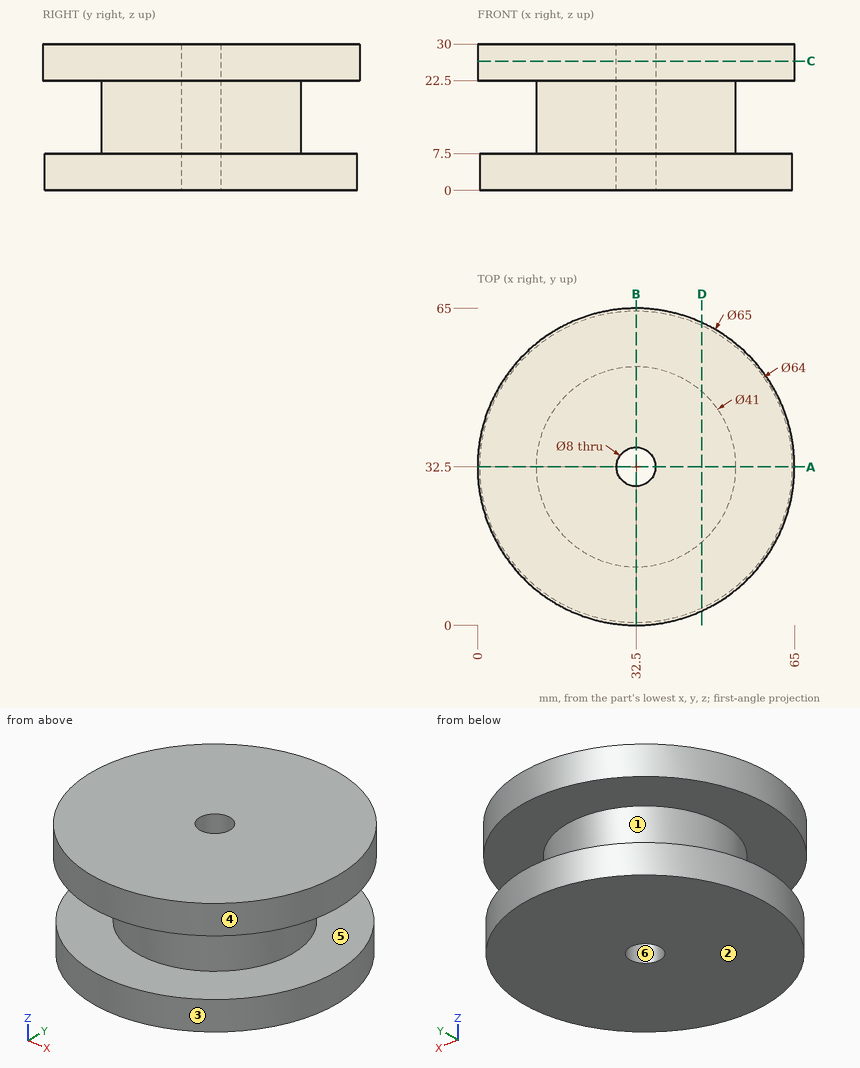
For this review, use the dimensioned drawing (mm, ordinates from the lowest corner) and the shaded views. A direction names the side the tool comes from. Give positions to 0.01 mm unless a question says otherwise; leave off trailing zeros. Order: outer loops, then holes, each group sorted by start corner. A loop starts at its lowest first (then second) coordinate and runs counter-clockwise, first axis right, second up. Notation, with made-up numbers: (-10, 37.25) - (-6, 37.25) arc R14 ccw to (-6, 41.25) - close; hole circle Ø4 at (21, -17.5). An arc over 180 degrees is marked (long way). Write item = value, one per line. Start each with the question number.
Q1. We need section A-A on y = 32.5. State the section outline as (x, z) points.
Q2. To check wall thickness, follow L1, parallel to Z at x = 11, y = 23.5; L2, parallel to Y at x = 32.5, z = 11.75; L3, parallel to Z at x = 19.5, y = 62. State the ranges of each line that lie inside material, in increasing order. Write a range as from..to.
Q3. We need section D-D on x = 46. State the section outline as (y, z) points.
Q4. We need section C-C on z = 26.5. State the section outline as (x, y) points, plus the area to 3 significant figures.
Q5. Clearance check with flat-ended pins moving along their axes: pin 1 Ø3 at (x, z) = (53.5, 24) entering from -Y; pin 2 Ø12 at (x, z) = (16.5, 19.5) entering from +Y; pin 3 Ø2 at (y, z) = (20, 4) entering from +X; pin 4 Ø10 at (x, y) = (45, 17.5) entering from -Z. State where each tip first meets the part, or that it passes through.
Q6. Tool access review of the marked faces 1, 2 and 3: name each direction out of +Z, -Z, +X, -X, +Y, -Y from which nothing blocks a thin tool from reaching the whole face with its end or side.
Q7. Mouldability with a two-part tool opening along X and no side actions: class the marked faces 4, 5 and 6 as released by +X, released by -X, zero draft, split by the parting line, or undercut.
Working result:
q1.outline = (0, 22.5) - (12, 22.5) - (12, 7.5) - (0.5, 7.5) - (0.5, 0) - (28.5, 0) - (28.5, 30) - (0, 30) - close; (36.5, 0) - (64.5, 0) - (64.5, 7.5) - (53, 7.5) - (53, 22.5) - (65, 22.5) - (65, 30) - (36.5, 30) - close
q2.L1 = 0..7.5, 22.5..30
q2.L2 = 12..28.5, 36.5..53
q2.L3 = 22.5..30
q3.outline = (2.94, 22.5) - (17.07, 22.5) - (17.07, 7.5) - (3.49, 7.5) - (3.49, 0) - (61.51, 0) - (61.51, 7.5) - (47.93, 7.5) - (47.93, 22.5) - (62.06, 22.5) - (62.06, 30) - (2.94, 30) - close
q4.outline = circle Ø65 at (32.5, 32.5); hole circle Ø8 at (32.5, 32.5)
q4.area = 3,270 mm²
q5.pin_1 = 6.5
q5.pin_2 = 63.15
q5.pin_3 = 62.36
q5.pin_4 = 0
q6.face_1 = none
q6.face_2 = -Z, +X, -X, +Y, -Y
q6.face_3 = -Z
q7.face_4 = split by the parting line
q7.face_5 = zero draft
q7.face_6 = undercut
